The model under review builds one solid part; all positions refer to its coordinate system, in mm. Face numbers are marked on the shaded views. Coordinates: 2 decimals unless noted, no trailing zeros. Write each loop counter-clockwise with the first axis right and the second up, starting at its lowest first coordinate (ties: lowest second). Pieces come first, ordered by that corner, then holes.
1) Mouldability with a two-part tool opening along X and no side actions: class the marked faces 1, 2 and 3 as released by +X, released by -X, zero draft, split by the parting line, or undercut.
2) Add section B-B, the plane z = 33. State the section outline as (x, y) points, then the cut area to 3 significant figures.
3) Add section D-D, the plane x = 20.5. State the section outline as (y, z) points, then the cut area to 3 significant figures.
4) For P1, Ø6.5, axis at x = 60, z = 0, coming from the +Y side; P2, Ø5, axis at x = 1.5, y = 164, coming from the -Z side; P3, Ø1, axis at y = 163, z = 29, coming from the +X side; P4, Ø2, axis at x = 28, y = 78.5, coming from the -Z side, all flat-tipped, find the tip position at first contact; note any pin that passes through.
5) Add section C-C, the plane y = 34. State the section outline as (x, z) points, then the cut area to 3 significant figures.
6) Add section A-A, the plane x = -60. State the section outline as (y, z) points (3 decimals), then the cut area to 3 significant figures.
7) For line 1 (X direction, y = 85, z = 0); line 2 (X direction, y = 107.5, z = -14.5); line 3 (Z direction, x = -12.5, y = 40), list the stretches that pass through material, from the lowest coordinate up.
from build123d import *

# Parameters (mm, degrees)
SKETCH_1_W               = 70
SKETCH_1_H               = 8
M8X1_0_2_D               = 8
M8X1_0_2_CSINK_D         = 8.05
M8X1_0_2_CSINK_ANGLE     = 100
PATTERN_CIRCULAR_2_COUNT = 8
SKETCH_11_W              = 50
SKETCH_11_H              = 190
SKETCH_12_R              = 45
CUT_EXTRUDE_1_DEPTH      = 222.368471106


with BuildPart() as part:
    # Sketch 1 → Revolve 1 (revolve)
    with BuildSketch(Plane.XY, mode=Mode.PRIVATE) as revolve_1_sk:
        with Locations((-35, 4)):
            Rectangle(SKETCH_1_W, SKETCH_1_H)
    revolve(revolve_1_sk.sketch.rotate(Axis((0, 76.619497233, 0), (0, -1, 0)), 270), axis=Axis((0, 76.619497233, 0), (0, -1, 0)))

    # M8x1.0 _2 (through all)
    with Locations(Plane(origin=(0, 8, 0), x_dir=(1, 0, 0), z_dir=(0, 1, 0))):
        with Locations((-60, 0)):
            m8x1_0_2 = CounterSinkHole(M8X1_0_2_D / 2, M8X1_0_2_CSINK_D / 2, counter_sink_angle=M8X1_0_2_CSINK_ANGLE)

    # Pattern Circular 2: M8x1.0 _2 ×8 about axis
    pattern_circular_2_axis = Axis((0, 0, 0), (0, 1, 0))
    for i in range(1, PATTERN_CIRCULAR_2_COUNT):
        add(m8x1_0_2.rotate(pattern_circular_2_axis, i * 360 / PATTERN_CIRCULAR_2_COUNT), mode=Mode.SUBTRACT)

    # Sketch 11 → Revolve 2 (revolve)
    with BuildSketch(Plane.XY, mode=Mode.PRIVATE) as revolve_2_sk:
        with Locations((-25, 103)):
            Rectangle(SKETCH_11_W, SKETCH_11_H)
    revolve(revolve_2_sk.sketch.rotate(Axis((0, 8, 0), (0, 1, 0)), 270), axis=Axis((0, 8, 0), (0, 1, 0)))

    # Sketch 12 → Cut-Extrude 1 (cut, through all)
    with BuildSketch(Plane.XZ):
        with Locations(Location((0, 0, 0), (0, 0, 270))):
            Circle(SKETCH_12_R)
    extrude(amount=-CUT_EXTRUDE_1_DEPTH, mode=Mode.SUBTRACT)


solid = part.part
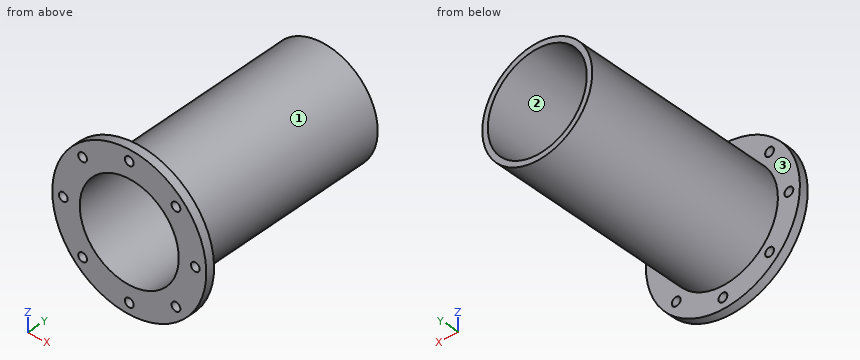
Geometry results:
1. face 1: split by the parting line
1. face 2: undercut
1. face 3: zero draft
2. outline: (-61.73, 0) - (-30.59, 0) - (-30.59, 198) - (-37.56, 198) - (-37.56, 8) - (-61.73, 8) - close; (30.59, 0) - (61.73, 0) - (61.73, 8) - (37.56, 8) - (37.56, 198) - (30.59, 198) - close
2. area: 3,150 mm2
3. outline: (0, -66.93) - (8, -66.93) - (8, -45.6) - (198, -45.6) - (198, -40.06) - (0, -40.06) - close; (0, 40.06) - (198, 40.06) - (198, 45.6) - (8, 45.6) - (8, 66.93) - (0, 66.93) - close
3. area: 2,540 mm2
4. P1: passes through
4. P2: stops at z = -50
4. P3: stops at x = 41.08
4. P4: stops at z = -42.08
5. outline: circle Ø100 at (0, 0); hole circle Ø90 at (0, 0)
5. area: 1,490 mm2
6. outline: (0, -36.056) - (8, -36.056) - (8, -4.025) - (7.979, -4) - (0, -4) - close; (0, 4) - (7.979, 4) - (8, 4.025) - (8, 36.056) - (0, 36.056) - close
6. area: 513 mm2
7. line 1: x = -50 to -45, 45 to 50
7. line 2: x = -47.85 to -42.6, 42.6 to 47.85
7. line 3: z = -48.41 to -43.23, 43.23 to 48.41
